Verification items for the finished model (mm, model axes). Face numbers are marked on the shaded views. A direction names the side the tool comes from. Round coordinates to 2 decimals unless told otherwise and drop trailing zeros. Write each loop counter-clockwise with the first axis right and the second up, starting at its lowest first coordinate (ties: lowest second). Pieces come first, ordered by that corner, then holes. Notation, with made-up numbers: (56.5, -36.75) - (109.5, -36.75) arc R4 cw to (109.5, -29.75) - close; hole circle Ø9 at (17.25, 54.5). An arc over 180 degrees is marked (long way). Answer as a JSON object with one key per item and string values. Group by question number.
1) Thickness scan on line 1 (Y direction, x = -16, z = 2.1) (3 decimals). Record the ranges inside material, lowest first.
2) Section check A-A (x = -16.5). Enter the section's corners in (y, z) (3 decimals), then the cut area to 3 significant figures.
3) Go/stop test with a flat-tipped pin: pin 1 Ø1.6 at (x, z) = (-17, 1) entering from +Y (3 decimals). Record where the tip stops, or that it passes through.
4) Set-up check for the marked faces 1 and 2: record each of +Z, -Z, +X, -X, +Y, -Y from which the full face is reachable in a straight line by a thin tool's end or side.
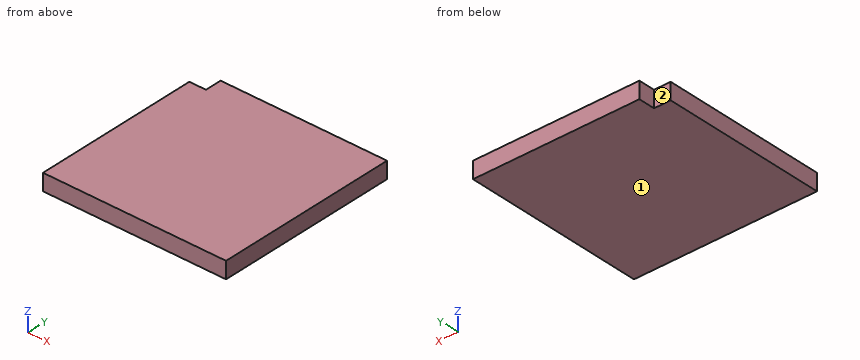
```python
from build123d import *

# Parameters (mm, degrees)
F0_W     = 31.75
F0_H     = 31.75
F1_DEPTH = 3.175
F2_W     = 31.75
F2_H     = 3.175
F3_DEPTH = 3.175
F4_W     = 3.175
F4_H     = 31.75
F5_DEPTH = 3.175


# Not quite as in the source:
# - a length typed as a fraction of an inch, garbled in the dataset ("3 / 203.2 mm" for 3/8 in), is restored


with BuildPart() as f1:
    # F0 (on Top) → F1 (new body)
    with BuildSketch(Plane.XY):
        Rectangle(F0_W, F0_H)
    extrude(amount=F1_DEPTH)

    # F2 (on face) → F3 (join)
    with BuildSketch(Plane.XY.offset(3.175)):
        with Locations((0, 17.4625)):
            Rectangle(F2_W, F2_H)
    extrude(amount=-F3_DEPTH)

    # F4 (on face) → F5 (join)
    with BuildSketch(Plane.XY.offset(3.175)):
        with Locations((-17.4625, 0)):
            Rectangle(F4_W, F4_H)
    extrude(amount=-F5_DEPTH)


solid = f1.part
```
Returned:
{
 "1": {"line 1": "-15.875 to 15.875"},
 "2": {"outline": "(-15.875, 0) - (15.875, 0) - (15.875, 3.175) - (-15.875, 3.175) - close", "area": "101 mm2"},
 "3": {"pin 1": "y = 15.875"},
 "4": {"face 1": "-Z, +X, -X, +Y, -Y", "face 2": "+Z, -Z, -X, +Y"}
}
